Work out the finished part from the listing and answer in its coordinate system (mm). Face numbers are marked on the shaded views. Round coordinates to 2 decimals unless told otherwise and drop trailing zeros. Loops run counter-clockwise (first coordinate to the right, second up) from the corner with the lowest first, then second, coordinate; pieces in that order, holes last. Notation, with made-up numbers: M -39.5,18.5 L -33.5,18.5 A22 cw -33.5,44.5 Z; hole C 10.5,-33.75 d2. An arc over 180 degrees is marked long. One line per item, written item: value.
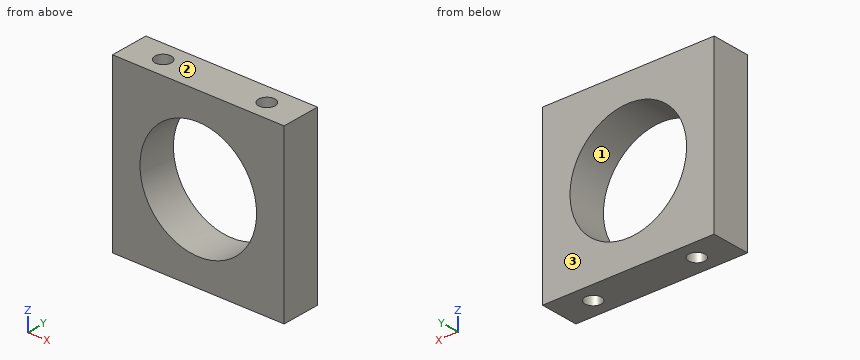
```python
from build123d import *

# Parameters (mm, degrees)
F0_W     = 42.0116
F0_H     = 42.0116
F0_R     = 14.2748
F1_DEPTH = 9.525
F2_R     = 2.0193
F3_DEPTH = 11.1125
F4_R     = 2.0193
F5_DEPTH = 11.1125


with BuildPart() as f1:
    # F0 (on Front) → F1 (new body)
    with BuildSketch(Plane.XZ):
        Rectangle(F0_W, F0_H)
        Circle(F0_R, mode=Mode.SUBTRACT)
    extrude(amount=F1_DEPTH)

    # F2 (on face) → F3 (cut)
    with BuildSketch(Plane.XY.offset(21.0058)):
        with Locations((-12.7, -4.7625)):
            Circle(F2_R)
        with Locations((12.7, -4.7625)):
            Circle(F2_R)
    extrude(amount=-F3_DEPTH, mode=Mode.SUBTRACT)

    # F4 (on face) → F5 (cut)
    with BuildSketch(Plane(origin=(0, 0, -21.0058), x_dir=(1, 0, 0), z_dir=(0, 0, -1))):
        with Locations((-12.7, 4.7625)):
            Circle(F4_R)
        with Locations((12.7, 4.7625)):
            Circle(F4_R)
    extrude(amount=-F5_DEPTH, mode=Mode.SUBTRACT)


solid = f1.part
```
1) The mould has two halves that part along Z. Classify the marked faces 1, 2 and 3: +Z half, -Z half, draft (parallel to the pull), parting line (faces both ways), or undercut.
Check values:
face 1: undercut
face 2: +Z half
face 3: draft
2) Find section D-D (y = -1.25). Give the vertices of the cut face in (x, z).
Check values:
outline: M -21.01,-21.01 L 21.01,-21.01 L 21.01,21.01 L -21.01,21.01 Z; hole C 0,0 d28.55
3) Find section C-C (z = 0). Give the vertices of the cut face in (x, y) (3 decimals).
Check values:
outline: M -21.006,-9.525 L -14.275,-9.525 L -14.275,0 L -21.006,0 Z; M 14.275,-9.525 L 21.006,-9.525 L 21.006,0 L 14.275,0 Z
4) Each of these flat-tipped pins is pushed along its axis until it touches: pin 1 (2.5 mm diameter, centred on x = 12.7, y = -4.76, fed in from -Z); pin 2 (3 mm diameter, centred on x = -13, y = -5, fed in from +Z). Where does it stop, or does it pass through?
Check values:
pin 1: z = -9.89
pin 2: z = 9.89
5) Find section B-B (z = 12). Give the vertices of the cut face in (x, y) (1 decimal), then the cut area to 3 significant figures.
Check values:
outline: M -21,-9.5 L -7.7,-9.5 L -7.7,0 L -21,0 Z; M 7.7,-9.5 L 21,-9.5 L 21,0 L 7.7,0 Z; hole C -12.7,-4.8 d4; hole C 12.7,-4.8 d4
area: 227 mm2
6) Find the intervals of material crossed by probe 1 along Y at (x, z) = (-12.7, 17.5) (3 decimals); probe 2 along Z at (x, y) = (-0.5, -2.25); probe 3 along X at (y, z) = (-6.5, -18), in increasing order. Write a range as from..to.
Check values:
probe 1: -9.525..-6.782, -2.743..0
probe 2: -21.01..-14.27, 14.27..21.01
probe 3: -21.01..-13.73, -11.67..11.67, 13.73..21.01
7) Find section A-A (x = 0). Give the vertices of the cut face in (y, z) (3 decimals), then the cut area to 3 significant figures.
Check values:
outline: M -9.525,-21.006 L 0,-21.006 L 0,-14.275 L -9.525,-14.275 Z; M -9.525,14.275 L 0,14.275 L 0,21.006 L -9.525,21.006 Z
area: 128 mm2
